```python
from build123d import *

# Parameters (mm, degrees)
SKETCH1_W           = 32.142857142
SKETCH1_H           = 6.35
SKETCH1_W_2         = 32.142857143
SKETCH1_W_3         = 6.35
SKETCH1_H_2         = 8.242857143
SKETCH1_H_3         = 8.242857142
BOSS_EXTRUDE1_DEPTH = 6.35
SKETCH2_W           = 212.3
SKETCH2_H           = 6.35
SKETCH2_W_2         = 5.08
BOSS_EXTRUDE2_DEPTH = 6.35
SKETCH3_W           = 35
SKETCH3_H           = 23.85
CUT_EXTRUDE1_DEPTH  = 235.025052078
SKETCH4_W           = 14.71
SKETCH4_H           = 6.35
SKETCH4_W_2         = 20.32
CUT_EXTRUDE2_DEPTH  = 6.35
SKETCH5_W           = 20.32
SKETCH5_H           = 6.35
SKETCH5_W_2         = 18.06
CUT_EXTRUDE3_DEPTH  = 235.025052078


with BuildPart() as part:
    # Sketch1 → Boss-Extrude1 (new body)
    with BuildSketch(Plane(origin=(0, 0, 0), x_dir=(1, 0, 0), z_dir=(0, 1, 0))):
        Polygon((6.35, 6.35), (32.142857143, 6.35), (64.285714286, 6.35), (96.428571429, 6.35), (128.571428571, 6.35), (160.714285714, 6.35), (192.857142857, 6.35), (218.65, 6.35), (218.65, 8.242857143), (218.65, 16.485714286), (218.65, 24.728571429), (218.65, 32.971428571), (218.65, 41.214285714), (218.65, 49.457142857), (218.65, 51.35), (192.857142857, 51.35), (160.714285714, 51.35), (128.571428571, 51.35), (96.428571429, 51.35), (64.285714286, 51.35), (32.142857143, 51.35), (6.35, 51.35), (6.35, 49.457142857), (6.35, 41.214285714), (6.35, 32.971428571), (6.35, 24.728571429), (6.35, 16.485714286), (6.35, 8.242857143), align=None)
        with Locations((112.5, 54.525)):
            Rectangle(SKETCH1_W, SKETCH1_H)
        with Locations((112.5, 3.175)):
            Rectangle(SKETCH1_W, SKETCH1_H)
        with Locations((176.785714286, 3.175)):
            Rectangle(SKETCH1_W_2, SKETCH1_H)
        with Locations((176.785714286, 54.525)):
            Rectangle(SKETCH1_W_2, SKETCH1_H)
        with Locations((48.214285715, 54.525)):
            Rectangle(SKETCH1_W_2, SKETCH1_H)
        with Locations((48.214285715, 3.175)):
            Rectangle(SKETCH1_W_2, SKETCH1_H)
        with Locations((3.175, 12.364285714)):
            Rectangle(SKETCH1_W_3, SKETCH1_H_2)
        with Locations((3.175, 28.85)):
            Rectangle(SKETCH1_W_3, SKETCH1_H_3)
        with Locations((3.175, 45.335714286)):
            Rectangle(SKETCH1_W_3, SKETCH1_H_2)
        with Locations((221.825, 12.364285714)):
            Rectangle(SKETCH1_W_3, SKETCH1_H_2)
        with Locations((221.825, 28.85)):
            Rectangle(SKETCH1_W_3, SKETCH1_H_3)
        with Locations((221.825, 45.335714286)):
            Rectangle(SKETCH1_W_3, SKETCH1_H_2)
    extrude(amount=BOSS_EXTRUDE1_DEPTH)

    # Sketch2 → Boss-Extrude2 (add)
    with BuildSketch(Plane(origin=(0, 6.35, 0), x_dir=(1, 0, 0), z_dir=(0, 1, 0))):
        with Locations((112.5, 54.525)):
            Rectangle(SKETCH2_W, SKETCH2_H)
        with Locations((23.6, 60.875)):
            Rectangle(SKETCH2_W_2, SKETCH2_H)
        with Locations((49, 60.875)):
            Rectangle(SKETCH2_W_2, SKETCH2_H)
        with Locations((74.4, 60.875)):
            Rectangle(SKETCH2_W_2, SKETCH2_H)
        with Locations((99.8, 60.875)):
            Rectangle(SKETCH2_W_2, SKETCH2_H)
        with Locations((201.4, 60.875)):
            Rectangle(SKETCH2_W_2, SKETCH2_H)
        with Locations((176, 60.875)):
            Rectangle(SKETCH2_W_2, SKETCH2_H)
        with Locations((125.2, 60.875)):
            Rectangle(SKETCH2_W_2, SKETCH2_H)
        with Locations((150.6, 60.875)):
            Rectangle(SKETCH2_W_2, SKETCH2_H)
    extrude(amount=-BOSS_EXTRUDE2_DEPTH)

    # Sketch3 → Cut-Extrude1 (cut, through all)
    with BuildSketch(Plane(origin=(0, 6.35, 0), x_dir=(1, 0, 0), z_dir=(0, 1, 0))):
        with Locations((112.5, 52.125)):
            Rectangle(SKETCH3_W, SKETCH3_H)
    extrude(amount=-CUT_EXTRUDE1_DEPTH, mode=Mode.SUBTRACT)

    # Sketch4 → Cut-Extrude2 (cut)
    with BuildSketch(Plane(origin=(0, 6.35, 0), x_dir=(1, 0, 0), z_dir=(0, 1, 0))):
        with Locations((13.705, 54.525)):
            Rectangle(SKETCH4_W, SKETCH4_H)
        with Locations((36.3, 54.525)):
            Rectangle(SKETCH4_W_2, SKETCH4_H)
        with Locations((211.295, 54.525)):
            Rectangle(SKETCH4_W, SKETCH4_H)
        with Locations((188.7, 54.525)):
            Rectangle(SKETCH4_W_2, SKETCH4_H)
    extrude(amount=-CUT_EXTRUDE2_DEPTH, mode=Mode.SUBTRACT)

    # Sketch5 → Cut-Extrude3 (cut, through all)
    with BuildSketch(Plane(origin=(0, 6.35, 0), x_dir=(1, 0, 0), z_dir=(0, 1, 0))):
        with Locations((61.7, 54.525)):
            Rectangle(SKETCH5_W, SKETCH5_H)
        with Locations((85.97, 54.525)):
            Rectangle(SKETCH5_W_2, SKETCH5_H)
        with Locations((139.03, 54.525)):
            Rectangle(SKETCH5_W_2, SKETCH5_H)
        with Locations((163.3, 54.525)):
            Rectangle(SKETCH5_W, SKETCH5_H)
    extrude(amount=-CUT_EXTRUDE3_DEPTH, mode=Mode.SUBTRACT)


solid = part.part
```
Source: CAD feature listing. Evaluate the final solid. Frame: model axes, mm. A direction names the side the tool comes from. Coordinates: 2 decimals unless noted, no trailing zeros. Write each loop counter-clockwise with the first axis right and the second up, starting at its lowest first coordinate (ties: lowest second). Pieces come first, ordered by that corner, then holes. Notation, with made-up numbers: M 42.5,87 L 70.5,87 A32 ccw 70.5,126 Z; hole C -37.75,63 d11. An arc over 180 degrees is marked long. Answer as a JSON object with one key per item and string values.
1. Cut plane D-D on z = -36. Output: boundary loops of the cut face in (x, y), plus the area to 3 significant figures.
Evaluation:
{"outline": "M 6.35,0 L 218.65,0 L 218.65,6.35 L 6.35,6.35 Z", "area": "1,350 mm^2"}
2. Draft query along Z for faces 1 (the flat face through (128.571, 3, -3)), 2 (the flat face through (48, 3, 0)), 3 (the flat face through (112, 3, -40.2)), 4 (the flat face through (218.65, 3, -37)). Return one class per face: released by +Z, released by -Z, zero draft, split by the parting line, or undercut.
Evaluation:
{"face 1": "zero draft", "face 2": "released by +Z", "face 3": "released by -Z", "face 4": "undercut"}
3. Cut plane A-A on z = -47. Output: boundary loops of the cut face in (x, y).
Evaluation:
{"outline": "M 0,0 L 95,0 L 95,6.35 L 0,6.35 Z; M 130,0 L 225,0 L 225,6.35 L 130,6.35 Z"}
4. Access query for faces 5 (the flat face through (64.286, 3, -3)), 6 (the flat face through (222, 3, -49.457)), 7 (the flat face through (163, 3, -51.35)). Directions: +Z, -Z, +X, -X, +Y, -Y. A direction counts if a zero-diameter tool reaches every point of the face in a straight line with its end or side. Return the directions, or none.
Evaluation:
{"face 5": "+Z, +Y, -Y", "face 6": "-Z, +X, +Y, -Y", "face 7": "-Z, +Y, -Y"}
5. Contact query for flat-ended pins moving along their axis: P1, Ø3, axis at x = 16.5, y = 2.5, coming from the -Z side; P2, Ø2, axis at y = 4.5, z = -50.5, coming from the -X side; P3, Ø1.5, axis at x = 136, y = 1, coming from the +Z side. Output: stop coordinate, or through.
Evaluation:
{"P1": "z = -51.35", "P2": "x = 6.35", "P3": "z = -6.35"}
6. Cut plane B-B on z = -58.5. Output: boundary loops of the cut face in (x, y).
Evaluation:
{"outline": "M 21.06,0 L 26.14,0 L 26.14,6.35 L 21.06,6.35 Z; M 46.46,0 L 51.54,0 L 51.54,6.35 L 46.46,6.35 Z; M 71.86,0 L 76.94,0 L 76.94,6.35 L 71.86,6.35 Z; M 148.06,0 L 153.14,0 L 153.14,6.35 L 148.06,6.35 Z; M 173.46,0 L 178.54,0 L 178.54,6.35 L 173.46,6.35 Z; M 198.86,0 L 203.94,0 L 203.94,6.35 L 198.86,6.35 Z"}
7. Cut plane C-C on x = 111. Output: boundary loops of the cut face in (y, z), plus the area to 3 significant figures.
Evaluation:
{"outline": "M 0,-40.2 L 6.35,-40.2 L 6.35,0 L 0,0 Z", "area": "255 mm^2"}
8. Ray query, L1, parallel to X at y = 0.5, z = -55.5; L2, parallel to X at y = 1.5, z = -43.5; L3, parallel to Z at x = 19, y = 3. Return the intervals inside material, ascending.
Evaluation:
{"L1": "21.06 to 26.14, 46.46 to 51.54, 71.86 to 76.94, 148.06 to 153.14, 173.46 to 178.54, 198.86 to 203.94", "L2": "0 to 95, 130 to 225", "L3": "-51.35 to -6.35"}
